The model under review builds one solid part; all positions refer to its coordinate system, in mm. Face numbers are marked on the shaded views. A direction names the side the tool comes from. Give positions to 0.01 mm unless a question says otherwise; leave off trailing zeros. Order: outer loops, then holes, each group sorted by start corner. A loop starts at its lowest first (then second) coordinate and runs counter-clockwise, first axis right, second up. Notation, with made-up numbers: (-27, 3) - (-9, 3) arc R21 ccw to (-9, 30) - close; hole circle Ø1 at (12.5, 62.25). An arc over 180 degrees is marked (long way). Write item = value, one per line. Start each with the question number.
1. We need section C-C, the plane x = 68.5. Give the boundary of the cut face in (y, z), and give its area (3 significant figures).
2. For P1, Ø5, axis at x = -6.35, y = 25.4, coming from the -Z side; P2, Ø4, axis at x = -3, y = 11.5, coming from the -Z side; P3, Ø12, axis at x = 53, z = 60.5, coming from the -Y side; P4, Ø3, axis at x = -4, z = 8, coming from the -Y side, all flat-tipped, find the tip position at first contact; note any pin that passes through.
3. We need section D-D, the plane y = 12.7. Give the boundary of the cut face in (x, z).
4. Machinability: for the marked faces 1 and 2, which of the approach directions +Z, -Z, +X, -X, +Y, -Y give a long, thin tool a straight path to every point of the face, cutting with its end or side? Answer none if there is none.
5. We need section B-B, the plane z = 136. Give the boundary of the cut face in (x, y), and give its area (3 significant figures).
6. Mouldability with a two-part tool opening along Z and no side actions: class the marked faces 3, 4, 5 and 6 as pulls with the +Z half, pulls with the -Z half, needs draft (parallel to the pull), parting line crosses it, or undercut.
7. We need section A-A, the plane y = 23.5. Give the boundary of the cut face in (x, z).
8. Wall thickness on probe 1 along Z at (x, y) = (46, 26); probe 2 along Z at (x, y) = (-0.5, 8); probe 3 along Y at (x, z) = (-6.35, 141): over which ranges is each line inside the solid? List them lowest first.
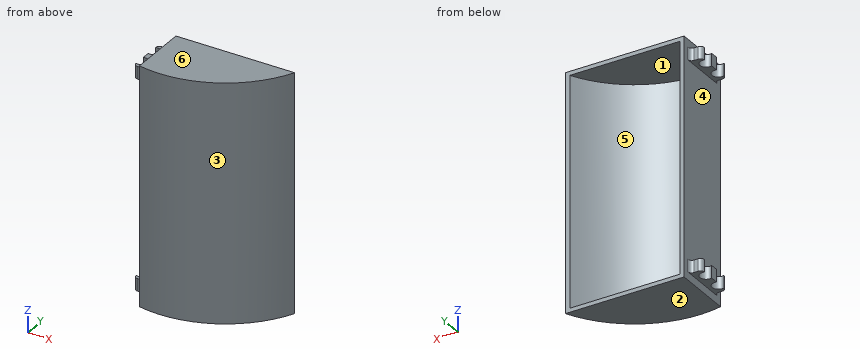
from build123d import *

# Parameters (mm, degrees)
BOSS_EXTRUDE1_DEPTH  = 152.4
SHELL1_T             = -2.54
SKETCH2_W            = 7.9375
SKETCH2_H            = 25.4
BOSS_EXTRUDE2_DEPTH  = 7.62
SKETCH3_R            = 3.9624
CUT_EXTRUDE1_DEPTH   = 12.7
FILLET1_R            = 2.54
FILLET1_OF_MIRROR1_R = 2.54


with BuildPart() as part:
    # Sketch1 → Boss-Extrude1 (new body)
    with BuildSketch(Plane.XY):
        with BuildLine():
            Line((0, 0), (0, 38.1))
            Line((0, 38.1), (76.2, 38.1))
            ThreePointArc((76.2, 38.1), (44.733669489, 5.782661022), (0, 0))
        make_face()
    extrude(amount=BOSS_EXTRUDE1_DEPTH)

    # Shell1
    shell1_openings = [part.faces().sort_by_distance(p)[0] for p in [
        (38.1, 38.1, 76.2),
    ]]
    offset(amount=SHELL1_T, openings=shell1_openings, kind=Kind.INTERSECTION)

    # Sketch2 → Boss-Extrude2 (add)
    with BuildSketch(Plane(origin=(0, 0, 0), x_dir=(0, 0, -1), z_dir=(1, 0, 0))):
        with Locations((-9.11225, 19.05)):
            Rectangle(SKETCH2_W, SKETCH2_H)
    boss_extrude2 = extrude(amount=-BOSS_EXTRUDE2_DEPTH)

    # Sketch3 → Cut-Extrude1 (cut)
    with BuildSketch(Plane(origin=(0, 0, 5.1435), x_dir=(-1, 0, 0), z_dir=(0, 0, -1))):
        with Locations((6.35, 25.4)):
            Circle(SKETCH3_R)
        with Locations((6.35, 12.7)):
            Circle(SKETCH3_R)
    cut_extrude1 = extrude(amount=-CUT_EXTRUDE1_DEPTH, mode=Mode.SUBTRACT)

    # Fillet1
    fillet1_edges = [part.edges().sort_by_distance(p)[0] for p in [
        (-7.62, 6.35, 9.11225),
        (-7.62, 31.75, 9.11225),
        (0, 31.75, 9.11225),
        (0, 6.35, 9.11225),
    ]]
    fillet(fillet1_edges, radius=FILLET1_R)

    # Mirror1: Boss-Extrude2, Cut-Extrude1 across plane
    add(boss_extrude2.mirror(Plane(origin=(0, 0, 76.2), x_dir=(1, 0, 0), z_dir=(0, 0, -1))))
    add(cut_extrude1.mirror(Plane(origin=(0, 0, 76.2), x_dir=(1, 0, 0), z_dir=(0, 0, -1))), mode=Mode.SUBTRACT)

    # Fillet1 of Mirror1
    fillet1_of_mirror1_edges = [part.edges().sort_by_distance(p)[0] for p in [
        (-7.62, 6.35, 143.28775),
        (-7.62, 31.75, 143.28775),
        (0, 31.75, 143.28775),
        (0, 6.35, 143.28775),
    ]]
    fillet(fillet1_of_mirror1_edges, radius=FILLET1_OF_MIRROR1_R)


solid = part.part
Model answer:
q1.outline = (25.41, 0) - (38.1, 0) - (38.1, 2.54) - (29.73, 2.54) - (29.73, 149.86) - (38.1, 149.86) - (38.1, 152.4) - (25.41, 152.4) - close
q1.area = 701 mm2
q2.P1 = through
q2.P2 = 5.14
q2.P3 = 6.97
q2.P4 = 6.35
q3.outline = (-2.39, 5.14) - (0, 5.14) - (0, 0) - (55.79, 0) - (55.79, 152.4) - (0, 152.4) - (0, 147.26) - (-2.39, 147.26) - (-2.39, 139.32) - (0, 139.32) - (0, 13.08) - (-2.39, 13.08) - close; hole (2.54, 2.54) - (51.47, 2.54) - (51.47, 149.86) - (2.54, 149.86) - close
q4.face_1 = +Y
q4.face_2 = -Z, +X, -X, +Y, -Y
q5.outline = (0, 0) arc R68.58 ccw to (76.2, 38.1) - (73.38, 38.1) arc R66.04 cw to (2.54, 2.1) - (2.54, 38.1) - (0, 38.1) - close
q5.area = 319 mm2
q6.face_3 = needs draft
q6.face_4 = undercut
q6.face_5 = undercut
q6.face_6 = pulls with the +Z half
q7.outline = (-2.87, 5.14) - (0, 5.14) - (0, 0) - (66.98, 0) - (66.98, 152.4) - (0, 152.4) - (0, 147.26) - (-2.87, 147.26) - (-2.87, 139.32) - (0, 139.32) - (0, 13.08) - (-2.87, 13.08) - close; hole (2.54, 2.54) - (63.65, 2.54) - (63.65, 149.86) - (2.54, 149.86) - close
q8.probe_1 = 0 to 2.54, 149.86 to 152.4
q8.probe_2 = 5.14 to 13.08, 139.32 to 147.26
q8.probe_3 = 6.69 to 8.74, 16.66 to 21.44, 29.36 to 31.41
